from build123d import *

# Parameters (mm, degrees)
SKETCH1_W           = 28
SKETCH1_H           = 10
SKETCH1_W_2         = 13.5
SKETCH1_H_2         = 24
BOSS_EXTRUDE1_DEPTH = 1
SKETCH2_W           = 14.5
SKETCH2_H           = 16.7
BOSS_EXTRUDE2_DEPTH = 15
SKETCH3_W           = 13.1
SKETCH3_H           = 5.74
CUT_EXTRUDE1_DEPTH  = 10
SKETCH4_W           = 7.814614209
SKETCH4_H           = 2.930480328
SKETCH4_H_2         = 2.083897123
BOSS_EXTRUDE3_DEPTH = 0.2


with BuildPart() as part:
    # Sketch1 → Boss-Extrude1 (new body)
    with BuildSketch(Plane(origin=(0, 0, 0), x_dir=(1, 0, 0), z_dir=(0, 1, 0))):
        Polygon((-4.896995708, 15.74248927), (8.603004292, 15.74248927), (15.853004292, 1.74248927), (-12.146995708, 1.74248927), align=None)
        with Locations((1.853004292, -3.25751073)):
            Rectangle(SKETCH1_W, SKETCH1_H)
        with Locations((1.853004292, 27.74248927)):
            Rectangle(SKETCH1_W_2, SKETCH1_H_2)
    extrude(amount=BOSS_EXTRUDE1_DEPTH)

    # Sketch2 → Boss-Extrude2 (add)
    with BuildSketch(Plane(origin=(0, 11, 0), x_dir=(1, 0, 0), z_dir=(0, 1, 0))):
        with Locations((1.853004292, -10.80751073)):
            Rectangle(SKETCH2_W, SKETCH2_H)
    extrude(amount=-BOSS_EXTRUDE2_DEPTH)

    # Sketch3 → Cut-Extrude1 (cut)
    with BuildSketch(Plane.XY.offset(19.15751073)):
        with Locations((1.816567827, 7.380781329)):
            Rectangle(SKETCH3_W, SKETCH3_H)
        with Locations((1.867135477, -0.457204484)):
            Rectangle(SKETCH3_W, SKETCH3_H)
    extrude(amount=-CUT_EXTRUDE1_DEPTH, mode=Mode.SUBTRACT)

    # Sketch4 → Boss-Extrude3 (add)
    with BuildSketch(Plane(origin=(0, 1, 0), x_dir=(1, 0, 0), z_dir=(0, 1, 0))):
        with Locations((1.885565184, 15.692844408)):
            Rectangle(SKETCH4_W, SKETCH4_H)
        with Locations((1.885565184, 38.257542937)):
            Rectangle(SKETCH4_W, SKETCH4_H_2)
    extrude(amount=BOSS_EXTRUDE3_DEPTH)


solid = part.part
Source: CAD feature listing. Evaluate the final solid. Frame: model axes, mm. A direction names the side the tool comes from. Coordinates: 2 decimals unless noted, no trailing zeros. Loops run counter-clockwise (first coordinate to the right, second up) from the corner with the lowest first, then second, coordinate; pieces in that order, holes last. Notation, with made-up numbers: (52.25, 33.5) - (103.25, 33.5) arc R31 ccw to (103.25, 58.5) - close; hole circle Ø2 at (16.25, 40). An arc over 180 degrees is marked (long way). Return JSON: item names as keys, results as strings.
Q1. Mould query, pull axis X, two halves, no side actions, for faces 4 (the flat face through (12.2, 0.5, -8.8)), 5 (the flat face through (-8.573, 0.493, -8.644)), 6 (the flat face through (2, 10.251, 14)), 7 (the flat face through (2, 6, 2.458)). Classes: released by +X, released by -X, zero draft, split by the parting line, or undercut.
Results:
{"face 4": "released by +X", "face 5": "released by -X", "face 6": "undercut", "face 7": "zero draft"}
Q2. Material intervals for line 1 along Y through (x, z) = (-4.75, -5); line 2 along Z through (x, y) = (-4.5, 0.75); line 3 along Z through (x, y) = (4.5, 2.75), sorted ascending.
Results:
{"line 1": "0 to 1", "line 2": "-39.74 to 9.16", "line 3": "2.46 to 19.16"}
Q3. Contact query for flat-ended pins moving along their axis: P1, Ø12, axis at x = 7, z = -6.5, coming from the +Y side; P2, Ø1.5, axis at x = 1, y = 7.5, coming from the -Z side; P3, Ø1.1, axis at x = -7.5, y = 0.5, coming from the +Z side. Output: stop coordinate, or through.
Results:
{"P1": "y = 1", "P2": "z = 2.46", "P3": "z = 8.26"}
Q4. Section A-A, the plane z = 13. Return loops of the section in (x, y).
Results:
{"outline": "(-5.4, -4) - (9.1, -4) - (9.1, 11) - (-5.4, 11) - close; hole (-4.73, 4.51) - (8.37, 4.51) - (8.37, 10.25) - (-4.73, 10.25) - close; hole (-4.68, -3.33) - (8.42, -3.33) - (8.42, 2.41) - (-4.68, 2.41) - close"}
Q5. Section B-B, the plane y = -0.75. Return loops of the section in (x, z).
Results:
{"outline": "(-5.4, 2.46) - (9.1, 2.46) - (9.1, 19.16) - (8.42, 19.16) - (8.42, 9.16) - (-4.68, 9.16) - (-4.68, 19.16) - (-5.4, 19.16) - close"}
Q6. Section C-C, the plane x = 5.25. Return loops of the section in (y, z), plus the area to 3 significant figures.
Results:
{"outline": "(-4, 2.46) - (0, 2.46) - (0, -39.74) - (1, -39.74) - (1, -39.3) - (1.2, -39.3) - (1.2, -37.22) - (1, -37.22) - (1, -17.16) - (1.2, -17.16) - (1.2, -14.23) - (1, -14.23) - (1, 2.46) - (11, 2.46) - (11, 19.16) - (10.25, 19.16) - (10.25, 9.16) - (4.51, 9.16) - (4.51, 19.16) - (2.41, 19.16) - (2.41, 9.16) - (-3.33, 9.16) - (-3.33, 19.16) - (-4, 19.16) - close", "area": "179 mm2"}
Q7. Access query for faces 1 (the flat face through (2, -2, 2.458)), 2 (the flat face through (2, 1.2, -38)), 3 (the flat face through (2, 2.413, 14)). Directions: +Z, -Z, +X, -X, +Y, -Y. A direction counts if a zero-diameter tool reaches every point of the face in a straight line with its end or side. Return the directions, or none.
Results:
{"face 1": "-Z, +X, -X, -Y", "face 2": "-Z, +X, -X, +Y", "face 3": "+Z"}
Q8. Section D-D, the plane z = 4.5. Return loops of the section in (x, y).
Results:
{"outline": "(-12.15, 0) - (-5.4, 0) - (-5.4, -4) - (9.1, -4) - (9.1, 0) - (15.85, 0) - (15.85, 1) - (9.1, 1) - (9.1, 11) - (-5.4, 11) - (-5.4, 1) - (-12.15, 1) - close"}
